For this review, take the finished solid that the model builds, in its own axes (mm). Face numbers are marked on the shaded views. A direction names the side the tool comes from. Give positions to 0.01 mm unless a question says otherwise; leave off trailing zeros. Order: outer loops, then holes, each group sorted by start corner. A loop starts at its lowest first (then second) coordinate and runs counter-clockwise, first axis right, second up.
Item 1: Consider section D-D (z = 11). Give the boundary of the cut face in (x, y).
Item 2: Consider section C-C (y = 14). Give the boundary of the cut face in (x, z), plus the area to 3 significant figures.
Item 3: Consider section B-B (z = -8.5). Give the boundary of the cut face in (x, y).
Item 4: Consider section A-A (x = 0). Give the boundary of the cut face in (y, z), plus the area to 3 significant figures.
Item 5: For probe 1 along X at (y, z) = (1.2, 11); probe 2 along X at (y, z) = (0.6, -8.5); probe 3 along Y at (x, z) = (-3.5, 5.5), list the stretches that pass through material, from the lowest coordinate up.
Item 6: For P1, Ø8, axis at x = 15.25, z = 11, coming from the +Y side; P2, Ø4, axis at x = -15.25, y = 33.5, coming from the +Z side; P3, Ø1.5, axis at x = 7, z = -3.5, coming from the -Y side; P4, Ø6.5, axis at x = 0, y = 14, coming from the +Z side, all flat-tipped, find the tip position at first contact; note any pin that passes through.
Item 7: Machinability: for the marked faces 1 and 2, which of the approach directions +Z, -Z, +X, -X, +Y, -Y give a long, thin tool a straight path to every point of the face, cutting with its end or side? Answer none if there is none.
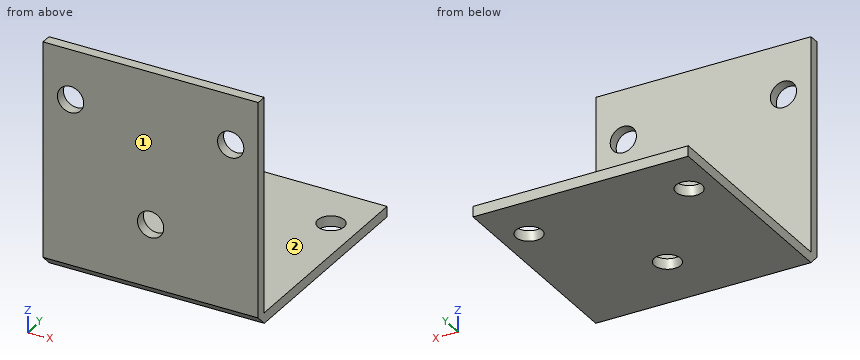
```python
from build123d import *

# Parameters (mm, degrees)
SKETCH_1_W          = 41
SKETCH_1_H          = 41
SKETCH_1_R          = 2.5
EXTRUDE_1_DEPTH     = 2
EXTRUDE_2_DEPTH     = 41
SKETCH_3_R          = 2.5
CUT_EXTRUDE_1_DEPTH = 3


with BuildPart() as part:
    # 草图1 → 凸台-拉伸1 (new body)
    with BuildSketch(Plane(origin=(0, 0, 0), x_dir=(1, 0, 0), z_dir=(0, 1, 0))):
        Rectangle(SKETCH_1_W, SKETCH_1_H)
        with Locations((-15.25, -11)):
            Circle(SKETCH_1_R, mode=Mode.SUBTRACT)
        with Locations((15.25, -11)):
            Circle(SKETCH_1_R, mode=Mode.SUBTRACT)
        with Locations((0, 8.5)):
            Circle(SKETCH_1_R, mode=Mode.SUBTRACT)
    extrude(amount=EXTRUDE_1_DEPTH)

    # 草图2 → 凸台-拉伸2 (add)
    with BuildSketch(Plane.ZY.offset(20.5)):
        Polygon((-22.5, 2), (-20.5, 0), (-20.5, 2), (-20.5, 43), (-22.5, 43), align=None)
    extrude(amount=-EXTRUDE_2_DEPTH)

    # 草图3 → 切除-拉伸1 (cut, through all)
    with BuildSketch(Plane.XY.offset(-20.5)):
        with Locations((-15.25, 33.5)):
            Circle(SKETCH_3_R)
        with Locations((15.25, 33.5)):
            Circle(SKETCH_3_R)
        with Locations((0, 14)):
            Circle(SKETCH_3_R)
    extrude(amount=-CUT_EXTRUDE_1_DEPTH, mode=Mode.SUBTRACT)


solid = part.part
```
Resolved:
1. outline: (-20.5, 0) - (-17.75, 0) - (-17.75, 2) - (-20.5, 2) - close; (-12.75, 0) - (12.75, 0) - (12.75, 2) - (-12.75, 2) - close; (17.75, 0) - (20.5, 0) - (20.5, 2) - (17.75, 2) - close
2. outline: (-20.5, -22.5) - (-2.5, -22.5) - (-2.5, -20.5) - (-20.5, -20.5) - close; (2.5, -22.5) - (20.5, -22.5) - (20.5, -20.5) - (2.5, -20.5) - close
2. area: 72.0 mm2
3. outline: (-20.5, 0) - (-2.5, 0) - (-2.5, 2) - (-20.5, 2) - close; (2.5, 0) - (20.5, 0) - (20.5, 2) - (2.5, 2) - close
4. outline: (0, -20.5) - (2, -22.5) - (11.5, -22.5) - (11.5, -20.5) - (2, -20.5) - (2, -11) - (0, -11) - close; (0, -6) - (2, -6) - (2, 20.5) - (0, 20.5) - close; (16.5, -22.5) - (43, -22.5) - (43, -20.5) - (16.5, -20.5) - close
4. area: 146 mm2
5. probe 1: x = -20.5 to -17.75, -12.75 to 12.75, 17.75 to 20.5
5. probe 2: x = -20.5 to -2.5, 2.5 to 20.5
5. probe 3: y = 0 to 2
6. P1: stops at y = 2
6. P2: passes through
6. P3: stops at y = 0
6. P4: stops at z = -20.5
7. face 1: +Z, -Z, +X, -X, -Y
7. face 2: +Z, +X, -X, +Y
